```python
from build123d import *

# Parameters (mm, degrees)
SKETCH_1_R      = 1.65
SKETCH_1_R_2    = 2.25
SKETCH_1_W      = 20
SKETCH_1_H      = 60
SKETCH_1_H_2    = 5
EXTRUDE_1_DEPTH = 2


with BuildPart() as part:
    # 草图1 → 凸台-拉伸1 (new body)
    with BuildSketch(Plane(origin=(0, 0, 0), x_dir=(1, 0, 0), z_dir=(0, 1, 0))):
        with BuildLine():
            Line((85, 50), (90, 50))
            ThreePointArc((90, 50), (97.071067812, 52.928932188), (100, 60))
            Line((100, 60), (100, 215))
            ThreePointArc((100, 215), (98.535533906, 218.535533906), (95, 220))
            Line((95, 220), (-95, 220))
            ThreePointArc((-95, 220), (-98.535533906, 218.535533906), (-100, 215))
            Line((-100, 215), (-100, 60))
            ThreePointArc((-100, 60), (-97.071067812, 52.928932188), (-90, 50))
            Line((-90, 50), (-85, 50))
            ThreePointArc((-85, 50), (-81.464466094, 48.535533906), (-80, 45))
            Line((-80, 45), (-80, -40))
            ThreePointArc((-80, -40), (-77.071067812, -47.071067812), (-70, -50))
            Line((-70, -50), (70, -50))
            ThreePointArc((70, -50), (77.071067812, -47.071067812), (80, -40))
            Line((80, -40), (80, 45))
            ThreePointArc((80, 45), (81.464466094, 48.535533906), (85, 50))
        make_face()
        with Locations(Location((47, -39.5, 0), (0, 0, 270))):
            Circle(SKETCH_1_R, mode=Mode.SUBTRACT)
        with Locations(Location((-40, 5, 0), (0, 0, 270))):
            Circle(SKETCH_1_R, mode=Mode.SUBTRACT)
        with Locations(Location((-40, -25, 0), (0, 0, 270))):
            Circle(SKETCH_1_R, mode=Mode.SUBTRACT)
        with Locations(Location((-70, -25, 0), (0, 0, 270))):
            Circle(SKETCH_1_R, mode=Mode.SUBTRACT)
        with Locations(Location((-70, 5, 0), (0, 0, 270))):
            Circle(SKETCH_1_R, mode=Mode.SUBTRACT)
        with Locations(Location((70, 5, 0), (0, 0, 270))):
            Circle(SKETCH_1_R, mode=Mode.SUBTRACT)
        with Locations(Location((70, -25, 0), (0, 0, 270))):
            Circle(SKETCH_1_R, mode=Mode.SUBTRACT)
        with Locations(Location((40, -25, 0), (0, 0, 270))):
            Circle(SKETCH_1_R, mode=Mode.SUBTRACT)
        with Locations(Location((40, 5, 0), (0, 0, 270))):
            Circle(SKETCH_1_R, mode=Mode.SUBTRACT)
        with Locations(Location((47, 24.5, 0), (0, 0, 270))):
            Circle(SKETCH_1_R, mode=Mode.SUBTRACT)
        with Locations(Location((15, 24.5, 0), (0, 0, 270))):
            Circle(SKETCH_1_R, mode=Mode.SUBTRACT)
        with Locations(Location((15, -39.5, 0), (0, 0, 270))):
            Circle(SKETCH_1_R, mode=Mode.SUBTRACT)
        with Locations(Location((-30.5, 76.5, 0), (0, 0, 270))):
            Circle(SKETCH_1_R, mode=Mode.SUBTRACT)
        with Locations(Location((-72.5, 76.5, 0), (0, 0, 270))):
            Circle(SKETCH_1_R, mode=Mode.SUBTRACT)
        with Locations(Location((-30.5, 17.5, 0), (0, 0, 270))):
            Circle(SKETCH_1_R, mode=Mode.SUBTRACT)
        with Locations(Location((-72.5, 17.5, 0), (0, 0, 270))):
            Circle(SKETCH_1_R, mode=Mode.SUBTRACT)
        with Locations(Location((22.5, 89.5, 0), (0, 0, 270))):
            Circle(SKETCH_1_R, mode=Mode.SUBTRACT)
        with Locations(Location((72.5, 89.5, 0), (0, 0, 270))):
            Circle(SKETCH_1_R, mode=Mode.SUBTRACT)
        with Locations(Location((72.5, 39.5, 0), (0, 0, 270))):
            Circle(SKETCH_1_R, mode=Mode.SUBTRACT)
        with Locations(Location((22.5, 39.5, 0), (0, 0, 270))):
            Circle(SKETCH_1_R, mode=Mode.SUBTRACT)
        with Locations(Location((0, 215, 0), (0, 0, 270))):
            Circle(SKETCH_1_R, mode=Mode.SUBTRACT)
        with Locations(Location((-85, 210, 0), (0, 0, 270))):
            Circle(SKETCH_1_R, mode=Mode.SUBTRACT)
        with Locations(Location((-55, 210, 0), (0, 0, 270))):
            Circle(SKETCH_1_R, mode=Mode.SUBTRACT)
        with Locations(Location((85, 210, 0), (0, 0, 270))):
            Circle(SKETCH_1_R, mode=Mode.SUBTRACT)
        with Locations(Location((55, 210, 0), (0, 0, 270))):
            Circle(SKETCH_1_R, mode=Mode.SUBTRACT)
        with Locations(Location((55, 160, 0), (0, 0, 270))):
            Circle(SKETCH_1_R, mode=Mode.SUBTRACT)
        with Locations(Location((0, 105, 0), (0, 0, 270))):
            Circle(SKETCH_1_R, mode=Mode.SUBTRACT)
        with Locations(Location((-55, 160, 0), (0, 0, 270))):
            Circle(SKETCH_1_R, mode=Mode.SUBTRACT)
        with Locations(Location((-55, -39.5, 0), (0, 0, 270))):
            Circle(SKETCH_1_R, mode=Mode.SUBTRACT)
        with Locations(Location((-20, 5.5, 0), (0, 0, 270))):
            Circle(SKETCH_1_R, mode=Mode.SUBTRACT)
        with Locations(Location((20, 5.5, 0), (0, 0, 270))):
            Circle(SKETCH_1_R, mode=Mode.SUBTRACT)
        with Locations(Location((0, 198.890872965, 0), (0, 0, 270))):
            Circle(SKETCH_1_R, mode=Mode.SUBTRACT)
        with Locations(Location((-38.890872965, 160, 0), (0, 0, 270))):
            Circle(SKETCH_1_R, mode=Mode.SUBTRACT)
        with Locations(Location((17.67766953, 103.431457505, 0), (0, 0, 270))):
            Circle(SKETCH_1_R, mode=Mode.SUBTRACT)
        with Locations(Location((56.568542495, 142.32233047, 0), (0, 0, 270))):
            Circle(SKETCH_1_R, mode=Mode.SUBTRACT)
        with Locations(Location((-21.5, 76.5, 0), (0, 0, 270))):
            Circle(SKETCH_1_R, mode=Mode.SUBTRACT)
        with Locations(Location((14.5, 76.5, 0), (0, 0, 270))):
            Circle(SKETCH_1_R, mode=Mode.SUBTRACT)
        with Locations(Location((14.5, 40.5, 0), (0, 0, 270))):
            Circle(SKETCH_1_R, mode=Mode.SUBTRACT)
        with Locations(Location((-21.5, 40.5, 0), (0, 0, 270))):
            Circle(SKETCH_1_R, mode=Mode.SUBTRACT)
        with Locations(Location((-91, 191, 0), (0, 0, 270))):
            Circle(SKETCH_1_R_2, mode=Mode.SUBTRACT)
        with Locations(Location((-91, 173, 0), (0, 0, 270))):
            Circle(SKETCH_1_R_2, mode=Mode.SUBTRACT)
        with Locations(Location((-59, 191, 0), (0, 0, 270))):
            Circle(SKETCH_1_R_2, mode=Mode.SUBTRACT)
        with Locations(Location((-59, 173, 0), (0, 0, 270))):
            Circle(SKETCH_1_R_2, mode=Mode.SUBTRACT)
        with Locations(Location((91, 191, 0), (0, 0, 270))):
            Circle(SKETCH_1_R_2, mode=Mode.SUBTRACT)
        with Locations(Location((59, 191, 0), (0, 0, 270))):
            Circle(SKETCH_1_R_2, mode=Mode.SUBTRACT)
        with Locations(Location((59, 173, 0), (0, 0, 270))):
            Circle(SKETCH_1_R_2, mode=Mode.SUBTRACT)
        with Locations(Location((91, 173, 0), (0, 0, 270))):
            Circle(SKETCH_1_R_2, mode=Mode.SUBTRACT)
        with Locations(Location((-40, 185, 0), (0, 0, 270))):
            Circle(SKETCH_1_R, mode=Mode.SUBTRACT)
        with Locations(Location((-40, 147, 0), (0, 0, 270))):
            Circle(SKETCH_1_R, mode=Mode.SUBTRACT)
        with Locations(Location((40, 147, 0), (0, 0, 270))):
            Circle(SKETCH_1_R, mode=Mode.SUBTRACT)
        with Locations(Location((40, 185, 0), (0, 0, 270))):
            Circle(SKETCH_1_R, mode=Mode.SUBTRACT)
        with Locations((75, 170)):
            Rectangle(SKETCH_1_W, SKETCH_1_H, mode=Mode.SUBTRACT)
        with BuildLine():
            Line((-28, -37.85), (-26, -37.85))
            ThreePointArc((-26, -37.85), (-24.35, -39.5), (-26, -41.15))
            Line((-26, -41.15), (-28, -41.15))
            ThreePointArc((-28, -41.15), (-29.65, -39.5), (-28, -37.85))
        make_face(mode=Mode.SUBTRACT)
        with Locations((75, 129.5)):
            Rectangle(SKETCH_1_W, SKETCH_1_H_2, mode=Mode.SUBTRACT)
        with Locations((-75, 170)):
            Rectangle(SKETCH_1_W, SKETCH_1_H, mode=Mode.SUBTRACT)
        with Locations((-75, 129.5)):
            Rectangle(SKETCH_1_W, SKETCH_1_H_2, mode=Mode.SUBTRACT)
    extrude(amount=EXTRUDE_1_DEPTH)


solid = part.part
```
Can you work these out from the model? Positions are in its coordinate system, mm. Coordinates: 2 decimals unless noted, no trailing zeros.
1. I need wall thicknesses on line 1 (Z direction, x = -59.5, y = 1.2); line 2 (Z direction, x = -70, y = 0.5); line 3 (X direction, y = 0.2, z = -182.5). Which ranges of each line are inside material? Lowest first, please.
2. I'm going to push a flat-ended pin straight in: pin 1 (1.5 mm diameter, centred on x = -55.5, z = -155, fed in from -Y). Where does the tip first touch, or does it pass through?
3. If we section it at A-A (y = 1.65): Give the number of separate pieces and of enclosed holes in the cut face, then the cut area to 3 significant figures.
Entries:
1. line 1: z = -220 to -193.19, -188.81 to -175.19, -170.81 to 50
1. line 2: z = -220 to -200, -140 to -132, -127 to -6.65, -3.35 to 23.35, 26.65 to 50
1. line 3: x = -100 to -85, -65 to 65, 85 to 100
2. pin 1: stops at y = 0
3. separate pieces: 1
3. enclosed holes: 56
3. area: 46,800 mm2
